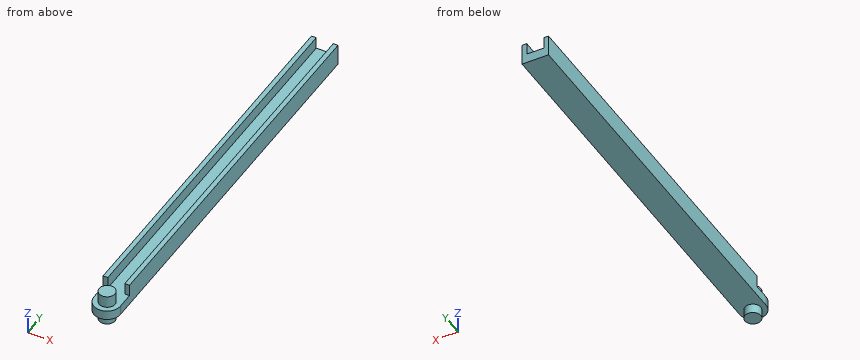
from build123d import *

# Parameters (mm, degrees)
SKETCH1_R      = 42.514793855
EXTRUDE1_DEPTH = 50.8
SKETCH1_4_W    = 25.4
SKETCH1_4_H    = 2018.826997117
EXTRUDE2_DEPTH = 114.3
EXTRUDE3_START = 50.8
SKETCH2_R      = 42.514793855
EXTRUDE3_DEPTH = 165.1


with BuildPart() as part:
    # Sketch1 → Extrude1 (new body)
    with BuildSketch(Plane.XY):
        with BuildLine():
            Line((-1183.595391403, 1195.645715897), (-1274.700151443, 1195.645715897))
            Line((-1274.700151443, 1195.645715897), (-1274.700151443, -823.18128122))
            Line((-1274.700151443, -823.18128122), (-1300.100151443, -823.18128122))
            Line((-1300.100151443, -823.18128122), (-1300.100151443, -911.736177467))
            ThreePointArc((-1300.100151443, -911.736177467), (-1229.147771423, -982.688557487), (-1158.195391403, -911.736177467))
            Line((-1158.195391403, -911.736177467), (-1158.195391403, -823.18128122))
            Line((-1158.195391403, -823.18128122), (-1183.595391403, -823.18128122))
            Line((-1183.595391403, -823.18128122), (-1183.595391403, 1195.645715897))
        make_face()
        with Locations((-1229.147771423, -911.736177467)):
            Circle(SKETCH1_R, mode=Mode.SUBTRACT)
    extrude(amount=EXTRUDE1_DEPTH)

    # Sketch1<4> → Extrude2 (add)
    with BuildSketch(Plane.XY):
        with Locations((-1287.400151443, 186.232217339)):
            Rectangle(SKETCH1_4_W, SKETCH1_4_H)
        with Locations((-1170.895391403, 186.232217339)):
            Rectangle(SKETCH1_4_W, SKETCH1_4_H)
    extrude(amount=EXTRUDE2_DEPTH)

    # Sketch2 → Extrude3 (add)
    with BuildSketch(Plane(origin=(0, 0, 0), x_dir=(-1, 0, 0), z_dir=(0, 0, -1)).offset(EXTRUDE3_START)):
        with Locations((1229.147771423, -911.736177467)):
            Circle(SKETCH2_R)
    extrude(amount=-EXTRUDE3_DEPTH)


solid = part.part
Work out the finished part from the listing and answer in its coordinate system (mm). Give positions to 0.01 mm unless a question says otherwise; leave off trailing zeros. Order: outer loops, then holes, each group sorted by start corner. A loop starts at its lowest first (then second) coordinate and runs counter-clockwise, first axis right, second up. Notation, with made-up numbers: (67, 67.5) -> (108, 67.5) arc R31 ccw to (108, 103.5) -> close; hole circle Ø9 at (-22.75, -39). An arc over 180 degrees is marked (long way). One line per item, written item: value.
Item 1: Straight lines are drawn through the part: probe 1 along X at (y, z) = (-319, 57.5); probe 2 along Z at (x, y) = (-1168.5, 665.5); probe 3 along Y at (x, z) = (-1228.5, 29). For each, find the intervals that lie inside material, in ascending order.
Answer sheet:
probe 1: -1300.1 to -1274.7, -1183.6 to -1158.2
probe 2: 0 to 114.3
probe 3: -982.69 to 1195.65
Item 2: Find section A-A, the plane y = 629.5. Give the vertices of the cut face in (x, z), plus the area to 3 significant figures.
Answer sheet:
outline: (-1300.1, 0) -> (-1158.2, 0) -> (-1158.2, 114.3) -> (-1183.6, 114.3) -> (-1183.6, 50.8) -> (-1274.7, 50.8) -> (-1274.7, 114.3) -> (-1300.1, 114.3) -> close
area: 10,400 mm²
Item 3: Flat-ended cylindrical pins translate along their axes: P1, Ø7.5, axis at x = -1165, z = 96, coming from the -Y side; P2, Ø1.5, axis at x = -1255.5, y = 308, coming from the +Z side; P3, Ø8, axis at x = -1228, y = 695, coming from the -Z side. Find the tip coordinate at first contact, or state that the pin passes through.
Answer sheet:
P1: y = -823.18
P2: z = 50.8
P3: z = 0
Item 4: Find section B-B, the plane x = -1225.5. Give the vertices of the cut face in (y, z).
Answer sheet:
outline: (-982.59, 0) -> (-954.09, 0) -> (-954.09, -50.8) -> (-869.38, -50.8) -> (-869.38, 0) -> (1195.65, 0) -> (1195.65, 50.8) -> (-869.38, 50.8) -> (-869.38, 114.3) -> (-954.09, 114.3) -> (-954.09, 50.8) -> (-982.59, 50.8) -> close
